Geometry check sheet. Reference: the model listing, model coordinates, mm. Face numbers are marked on the shaded views. Round coordinates to 2 decimals unless told otherwise and drop trailing zeros. Loops run counter-clockwise (first coordinate to the right, second up) from the corner with the lowest first, then second, coordinate; pieces in that order, holes last. Notation, with made-up numbers: M 84,26.5 L 95,26.5 A29 cw 95,54.5 Z; hole C -35,82.25 d10. An arc over 180 degrees is marked long. Answer in a Markdown table with one row per item. Add a question column.
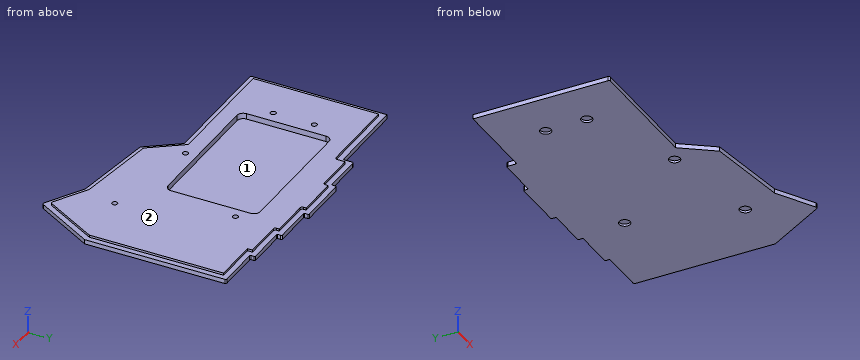
```python
from build123d import *

# Parameters (mm, degrees)
PAD022_DEPTH    = 2
PAD023_DEPTH    = 1
SKETCH097_R     = 1.25
POCKET015_DEPTH = 3.001
POCKET017_DEPTH = 2.6
SKETCH106_R     = 2.5
POCKET020_DEPTH = 1
SKETCH107_R     = 1.264414
SKETCH107_R_2   = 1.25
PAD027_DEPTH    = 0.24


with BuildPart() as part:
    # Sketch095 (on Face1 of ShapeBinder) → Pad022 (new body)
    with BuildSketch(Plane(origin=(0, 0, -16), x_dir=(1, 0, 0), z_dir=(0, 0, -1))):
        with BuildLine():
            Line((-2.2752, 3), (54.173381, 3))
            Line((54.173381, 3), (64.759843, 17.512342))
            Line((64.759843, 17.512342), (102.945986, 22.478633))
            Line((102.945986, 22.478633), (119.981121, 32.333705))
            ThreePointArc((121.153574, 32.019327), (120.632553, 32.419699), (119.981121, 32.333705))
            Line((121.153574, 32.019327), (136.73, 4.963884))
            Line((136.73, 4.963884), (136.73, -58.882076))
            ThreePointArc((136.112076, -59.5), (136.549014, -59.319014), (136.73, -58.882076))
            Line((136.112076, -59.5), (116.333806, -59.5))
            ThreePointArc((116.333806, -59.5), (116.083627, -59.603627), (115.98, -59.853806))
            Line((115.98, -59.853806), (115.98, -61.299282))
            ThreePointArc((115.529282, -61.75), (115.847988, -61.617988), (115.98, -61.299282))
            Line((115.529282, -61.75), (97.198754, -61.75))
            ThreePointArc((97.198754, -61.75), (97.044072, -61.814072), (96.98, -61.968754))
            Line((96.98, -61.968754), (96.98, -63.416556))
            ThreePointArc((96.396556, -64), (96.809113, -63.829113), (96.98, -63.416556))
            Line((96.396556, -64), (78.3317, -64))
            ThreePointArc((78.3317, -64), (78.083011, -64.103011), (77.98, -64.3517))
            Line((77.98, -64.3517), (77.98, -65.831599))
            ThreePointArc((77.561599, -66.25), (77.857453, -66.127453), (77.98, -65.831599))
            Line((77.561599, -66.25), (54.449571, -66.25))
            ThreePointArc((53.98, -65.780429), (54.117534, -66.112466), (54.449571, -66.25))
            Line((53.98, -65.780429), (53.98, -64.448303))
            ThreePointArc((53.98, -64.448303), (53.848695, -64.131305), (53.531697, -64))
            Line((53.531697, -64), (35.784272, -64))
            ThreePointArc((34.98, -63.195728), (35.215566, -63.764434), (35.784272, -64))
            Line((34.98, -63.195728), (34.98, -59.939901))
            ThreePointArc((34.98, -59.939901), (34.777933, -59.452067), (34.290099, -59.25))
            Line((34.290099, -59.25), (-3, -59.25))
            Line((-3, -59.25), (-3, 2.2752))
            ThreePointArc((-2.2752, 3), (-2.787711, 2.787711), (-3, 2.2752))
        make_face()
    extrude(amount=PAD022_DEPTH)

    # Sketch096 (on Face1 of ShapeBinder) → Pad023 (join)
    with BuildSketch(Plane(origin=(0, 0, -16), x_dir=(1, 0, 0), z_dir=(0, 0, -1))):
        with BuildLine():
            Line((-0.132, 0.5), (55.444173, 0.5))
            Line((55.444173, 0.5), (66.201245, 15.24622))
            Line((66.201245, 15.24622), (103.915077, 20.151085))
            Line((103.915077, 20.151085), (119.119523, 28.947076))
            ThreePointArc((120.320286, 28.621968), (119.787102, 29.032711), (119.119523, 28.947076))
            Line((120.320286, 28.621968), (134.23, 4.188169))
            Line((134.23, 4.188169), (134.23, -56.944054))
            ThreePointArc((134.174054, -57), (134.214403, -56.984403), (134.23, -56.944054))
            Line((134.174054, -57), (113.48, -57))
            Line((113.48, -57), (113.48, -59.216584))
            ThreePointArc((113.446584, -59.25), (113.470113, -59.240113), (113.48, -59.216584))
            Line((113.446584, -59.25), (95.423253, -59.25))
            ThreePointArc((95.423253, -59.25), (94.757913, -59.527912), (94.48, -60.193252))
            Line((94.48, -60.193252), (94.48, -61.412355))
            ThreePointArc((94.392355, -61.5), (94.454172, -61.474172), (94.48, -61.412355))
            Line((94.392355, -61.5), (76.471748, -61.5))
            ThreePointArc((76.471748, -61.5), (75.770092, -61.790091), (75.48, -62.491747))
            Line((75.48, -62.491747), (75.48, -63.721105))
            ThreePointArc((75.451105, -63.75), (75.471446, -63.741446), (75.48, -63.721105))
            Line((75.451105, -63.75), (56.567844, -63.75))
            ThreePointArc((56.48, -63.662156), (56.505729, -63.724271), (56.567844, -63.75))
            Line((56.48, -63.662156), (56.48, -62.563591))
            ThreePointArc((56.48, -62.563591), (56.168481, -61.811519), (55.416409, -61.5))
            Line((55.416409, -61.5), (37.73341, -61.5))
            ThreePointArc((37.48, -61.24659), (37.554222, -61.425778), (37.73341, -61.5))
            Line((37.48, -61.24659), (37.48, -58.013133))
            ThreePointArc((37.48, -58.013133), (37.110037, -57.119963), (36.216867, -56.75))
            Line((36.216867, -56.75), (-0.5, -56.75))
            Line((-0.5, -56.75), (-0.5, 0.132))
            ThreePointArc((-0.132, 0.5), (-0.392215, 0.392215), (-0.5, 0.132))
        make_face()
    extrude(amount=-PAD023_DEPTH)

    # Sketch097 → Pocket015 (cut, through all)
    with BuildSketch(Plane(origin=(0, 0, -18), x_dir=(1, 0, 0), z_dir=(0, 0, -1))):
        with Locations((18.61, -37.509997)):
            Circle(SKETCH097_R)
        with Locations((18.6, -18.76)):
            Circle(SKETCH097_R)
        with Locations((61.84, -1.51)):
            Circle(SKETCH097_R)
        with Locations((108.3, 6.24)):
            Circle(SKETCH097_R)
        with Locations((94.55, -41.5)):
            Circle(SKETCH097_R)
    extrude(amount=-POCKET015_DEPTH, mode=Mode.SUBTRACT)

    # Sketch100 → Pocket017 (cut)
    with BuildSketch(Plane.XY.offset(-15)):
        with BuildLine():
            Line((24.046659, 45.716233), (24.046659, 9.526233))
            ThreePointArc((24.046659, 9.526233), (24.897514, 7.472088), (26.951659, 6.621233))
            Line((26.951659, 6.621233), (86.530577, 6.621233))
            ThreePointArc((86.530577, 6.621233), (88.584722, 7.472088), (89.435577, 9.526233))
            Line((89.435577, 9.526233), (89.435577, 45.716233))
            ThreePointArc((89.435577, 45.716233), (88.584722, 47.770378), (86.530577, 48.621233))
            Line((86.530577, 48.621233), (26.951659, 48.621233))
            ThreePointArc((26.951659, 48.621233), (24.897514, 47.770378), (24.046659, 45.716233))
        make_face()
    extrude(amount=-POCKET017_DEPTH, mode=Mode.SUBTRACT)

    # Sketch106 (on Face5 of Pocket017) → Pocket020 (cut)
    with BuildSketch(Plane(origin=(0, 0, -18), x_dir=(1, 0, 0), z_dir=(0, 0, -1))):
        with Locations((61.84, -1.51)):
            Circle(SKETCH106_R)
        with Locations((108.3, 6.24)):
            Circle(SKETCH106_R)
        with Locations((94.55, -41.5)):
            Circle(SKETCH106_R)
        with Locations((18.61, -37.509997)):
            Circle(SKETCH106_R)
        with Locations((18.6, -18.76)):
            Circle(SKETCH106_R)
    extrude(amount=-POCKET020_DEPTH, mode=Mode.SUBTRACT)

    # Sketch107 (on Face70 of Pocket020) → Pad027 (join)
    with BuildSketch(Plane(origin=(0, 0, -17), x_dir=(1, 0, 0), z_dir=(0, 0, -1))):
        with Locations((61.84, -1.51)):
            Circle(SKETCH107_R)
        with Locations((18.6, -18.76)):
            Circle(SKETCH107_R_2)
        with Locations((108.3, 6.24)):
            Circle(SKETCH107_R_2)
        with Locations((94.55, -41.5)):
            Circle(SKETCH107_R_2)
        with Locations((18.61, -37.509997)):
            Circle(SKETCH107_R_2)
    extrude(amount=-PAD027_DEPTH)


with BuildPart() as part_1:
    # Body placement: moved
    add(part.part.moved(Location((0, 0, 9.4))))


solid = part_1.part
```
1) Cross-section at B-B, the plane x = 81.5. Record the boundary of the cut face in (y, z).
2) Thickness scan on L1, parallel to X at y = 18.76, z = -8.05; L2, parallel to Y at x = 18.6, z = -6.2; L3, parallel to X at y = 14, z = -6.4. Record the ranges inside material, lowest first. Write a range as [from, to].
3) Cross-section at A-A, the plane x = 45. Record the boundary of the cut face in (y, z), plus the area to 3 significant figures.
4) Go/stop test with flat-tipped pins: pin 1 (0.5 mm diameter, centred on y = 41, z = -6, fed in from -X); pin 2 (6 mm diameter, centred on x = 68.5, y = 19.5, fed in from +Z); pin 3 (0.6 mm diameter, centred on x = 88, z = -7.5, fed in from +Y). Record where each tip stops, or that it passes through.
5) Draft check along X on the marked faces 1 and 2. Enter one of: +X half, -X half, draft (parallel to the pull), parting line (faces both ways), or undercut.
Worked answers:
| question | item | result |
|---|---|---|
| 1 | outline | M -19.69,-8.6 L 64,-8.6 L 64,-6.6 L 61.5,-6.6 L 61.5,-5.6 L 48.62,-5.6 L 48.62,-8.2 L 6.62,-8.2 L 6.62,-5.6 L -17.24,-5.6 L -17.24,-6.6 L -19.69,-6.6 Z |
| 2 | L1 | x = [-3, 16.1], [21.1, 24.05], [89.44, 136.73] |
| 2 | L2 | y = [-0.5, 17.51], [20.01, 36.26], [38.76, 56.75] |
| 2 | L3 | x = [-0.5, 24.05], [89.44, 134.23] |
| 3 | outline | M -3,-8.6 L 64,-8.6 L 64,-6.6 L 61.5,-6.6 L 61.5,-5.6 L 48.62,-5.6 L 48.62,-8.2 L 6.62,-8.2 L 6.62,-5.6 L -0.5,-5.6 L -0.5,-6.6 L -3,-6.6 Z |
| 3 | area | 86.8 mm2 |
| 4 | pin 1 | stops at x = -0.5 |
| 4 | pin 2 | stops at z = -8.2 |
| 4 | pin 3 | stops at y = 64 |
| 5 | face 1 | undercut |
| 5 | face 2 | draft |
